CAD build for the part. Positions are in the model's coordinates, mm. Face numbers are marked on the shaded views. A direction names the side the tool comes from. Round coordinates to 2 decimals unless told otherwise and drop trailing zeros. Write each loop counter-clockwise with the first axis right and the second up, starting at its lowest first coordinate (ties: lowest second). Pieces come first, ordered by that corner, then holes. Notation, with made-up numbers: (9, 46) -> (21, 46) arc R16 ccw to (21, 76) -> close; hole circle Ø10 at (28.5, 83.5). An arc over 180 degrees is marked (long way). Put each result on its own line as item: value. Start each with the question number.
1. Saw through at B-B on y = -9.5. List the corners of the cut face in (x, z), and give its area (3 significant figures).
2. Drill centre lines: line 1 (Y direction, x = -2.75, z = 1.5); line 2 (Z direction, x = 2.5, y = -17.5); line 3 (Y direction, x = 3.5, z = 2.25). Where is each one in solid material? Low to high. Write a range as from..to.
3. 3-axis set-ups, long thin cutter, end or side, ignore diameter. For the marked faces 1 and 2: which of +Z, -Z, +X, -X, +Y, -Y reach the whole face in a straight line?
4. Saw through at A-A on y = -65.5. List the corners of the cut face in (x, z).
5. Flat gauge pins, fed straight in: P1, Ø1.5, axis at x = 1.5, y = -111, coming from the +Z side; P2, Ø1.5, axis at x = 2.5, y = -48, coming from the -Z side; P3, Ø1, axis at x = 3, y = -108.5, coming from the -Z side. Where does each tip first touch, or does it go through?
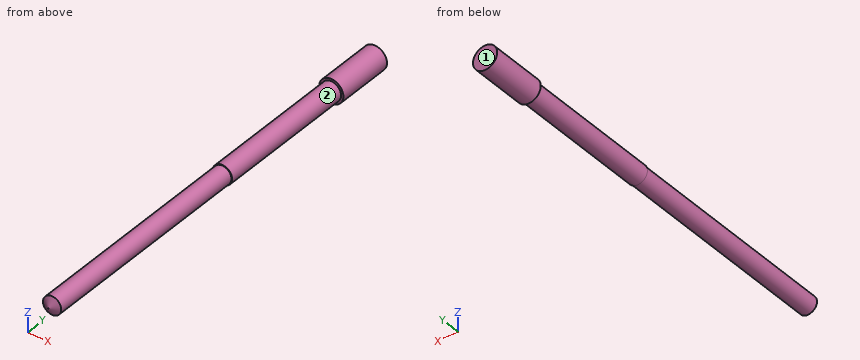
from build123d import *

# Parameters (mm, degrees)
F0_R     = 3.175
F1_DEPTH = 149.86
F2_SIZE2 = 3.048
F2_SIZE  = 1.7597636205
F3_R     = 3.4
F4_DEPTH = 70
F5_R     = 4.2017465395
F6_DEPTH = 20


with BuildPart() as f1:
    # F0 (on Front) → F1 (new body)
    with BuildSketch(Plane.XZ):
        Circle(F0_R)
    extrude(amount=F1_DEPTH)

    # F2
    f2_edges = [f1.edges().sort_by_distance(p)[0] for p in [
        (-3.175, -149.86, 0),
    ]]
    f2_side = f1.faces().sort_by_distance((-3.175, -74.93, 0))[0]
    chamfer(f2_edges, length=F2_SIZE, length2=F2_SIZE2, reference=f2_side)

    # F3 (on Front) → F4 (join)
    with BuildSketch(Plane.XZ):
        Circle(F3_R)
    extrude(amount=F4_DEPTH)

    # F5 (on Front) → F6 (join)
    with BuildSketch(Plane.XZ):
        Circle(F5_R)
    extrude(amount=F6_DEPTH)


solid = f1.part
Return value:
1. outline: circle Ø8.4 at (0, 0)
1. area: 55.5 mm^2
2. line 1: y = -148.12..0
2. line 2: z = -3.38..3.38
2. line 3: y = -20..0
3. face 1: +Z, -Z, +X, -X, +Y
3. face 2: -Y
4. outline: circle Ø6.8 at (0, 0)
5. P1: stops at z = 3.09
5. P2: stops at z = -2.92
5. P3: stops at z = -1.96
